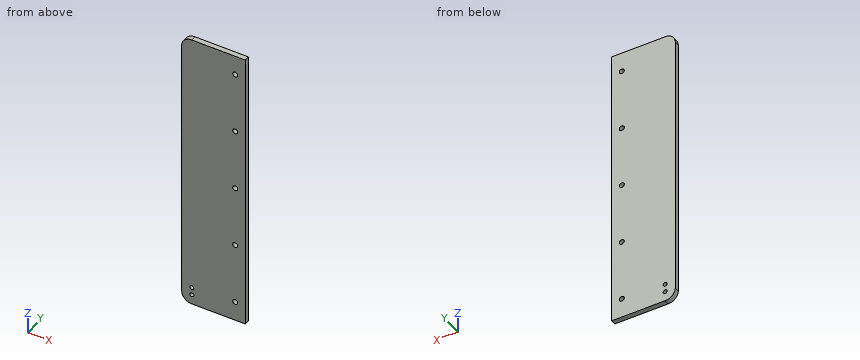
Autodesk Inventor part; units mm, degrees
ref_plane "YZ Plane" through (0, 0, 0) normal (1, 0, 0) x (0, 1, 0)
ref_plane "XZ Plane" through (0, 0, 0) normal (0, 1, 0) x (-1, 0, 0)
ref_plane "XY Plane" through (0, 0, 0) normal (0, 0, 1) x (1, 0, 0)
sketch "Sketch1" plane through (0, 0, 0) normal (0, 1, 0) x (-1, 0, 0)
  line L0 (0, 0) -> (63, 0)
  line L1 (63, 0) -> (63, -290)
  line L2 (63, -290) -> (0, -290)
  line L3 (0, -290) -> (0, 0)
  dimension "d0" = 290
  dimension "d1" = 63
extrude "Extrusion1" add sketch "Sketch1" along normal blind 5
fillet "Fillet1" radius 10 2 edges at (-63, 2.5, 0) (-63, 2.5, -290)
sketch "Sketch2" plane through (0, 0, 0) normal (0, -1, 0) x (1, 0, 0)
  line L0 (-53, -251.9925) -> (-53, -308.0075) construction
  line L1 (-63, -280) -> (-63, -10)
  circle A0 centre (-53, -280) radius 2
  circle A1 centre (-53, -272) radius 2
  line L2 (0, -290) -> (-53, -290)
  point P0 (0, 0)
  dimension "d5" = 10
  dimension "d6" = 4
  dimension "d7" = 4
  dimension "d8" = 8
  dimension "d9" = 10
hole "Hole1" at (-53, 0, -280) at (-53, 0, -272) direction (0, 1, 0) diameter 4 end through all
sketch "Sketch3" plane through (0, 5, 0) normal (0, 1, 0) x (1, 0, 0)
  line L0 (-10, -16.5573) -> (-10, 317.2677) construction
  line L1 (0, 0) -> (0, 290)
  circle A0 centre (-10, 20) radius 2.5
  circle A1 centre (-10, 270) radius 2.5
  circle A2 centre (-10, 82.5) radius 2.5
  circle A3 centre (-10, 145) radius 2.5
  line L2 (-53, 0) -> (0, 0)
  line L3 (0, 290) -> (-53, 290)
  circle A4 centre (-10, 207.5) radius 2.5
  dimension "d17" = 10
  dimension "d18" = 20
  dimension "d19" = 20
  dimension "d20" = 62.5
  dimension "d21" = 62.5
  dimension "d22" = 62.5
  dimension "d23" = 5
  dimension "d24" = 5
  dimension "d25" = 5
  dimension "d26" = 5
  dimension "d27" = 5
hole "Hole2" at (-10, 5, -20) at (-10, 5, -82.5) at (-10, 5, -145) at (-10, 5, -207.5) at (-10, 5, -270) direction (0, -1, 0) diameter 5 end through all
equation "\"d7\" = d6"
equation "\"d10\" = d6"
equation "\"d24\" = d23"
equation "\"d25\" = d24"
equation "\"d26\" = d25"
equation "\"d27\" = d26"
equation "\"d28\" = d23"
properties part number "Y_Kettenhalter"
Read the model definition and answer for the solid it produces. Units are mm, in the model's axes. Coordinates: 2 decimals unless noted, no trailing zeros. Write each loop counter-clockwise with the first axis right and the second up, starting at its lowest first coordinate (ties: lowest second). Pieces come first, ordered by that corner, then holes. Notation, with made-up numbers: M 19.5,-4.5 L 61.5,-4.5 A21 cw 61.5,13.5 Z; hole C 65,-6.5 d6. An arc over 180 degrees is marked long. Use a Markdown table: item, result.
Q1. Straight lines are drawn through the part: L1, parallel to Z at x = -53, y = 2; L2, parallel to Z at x = -10, y = 2; L3, parallel to X at y = 3.75, z = -82.5. For each, find the intervals that lie inside material, in ascending order. Write a range as [from, to].
Answer block:
| item | result |
|---|---|
| L1 | z = [-290, -282], [-278, -274], [-270, 0] |
| L2 | z = [-290, -272.5], [-267.5, -210], [-205, -147.5], [-142.5, -85], [-80, -22.5], [-17.5, 0] |
| L3 | x = [-63, -12.5], [-7.5, 0] |
Q2. The part is cut by section A-A, the plane z = -20. Write down the section's boundary in (x, y).
Answer block:
| item | result |
|---|---|
| outline | M -63,0 L -12.5,0 L -12.5,5 L -63,5 Z; M -7.5,0 L 0,0 L 0,5 L -7.5,5 Z |
Q3. The part is cut by section B-B, the plane x = -10. Write down the section's boundary in (y, z).
Answer block:
| item | result |
|---|---|
| outline | M 0,-290 L 5,-290 L 5,-272.5 L 0,-272.5 Z; M 0,-267.5 L 5,-267.5 L 5,-210 L 0,-210 Z; M 0,-205 L 5,-205 L 5,-147.5 L 0,-147.5 Z; M 0,-142.5 L 5,-142.5 L 5,-85 L 0,-85 Z; M 0,-80 L 5,-80 L 5,-22.5 L 0,-22.5 Z; M 0,-17.5 L 5,-17.5 L 5,0 L 0,0 Z |
